The figure shows three views and two pictorial views of one solid part (mm, origin at its lowest corner). Answer the questions. A direction names the side the tool comes from. Round coordinates to 2 decimals unless told otherwise and drop trailing zeros. Order: outer loops, then holes, each group sorted by start corner. A loop starts at its lowest first (then second) coordinate and runs counter-clockwise, first axis right, second up. Notation, with made-up numbers: (9, -15) - (66, -15) arc R32 ccw to (66, 16) - close; hole circle Ø8 at (-29, 33). An arc over 180 degrees is marked (long way). Answer in a Markdown table with one row per item.
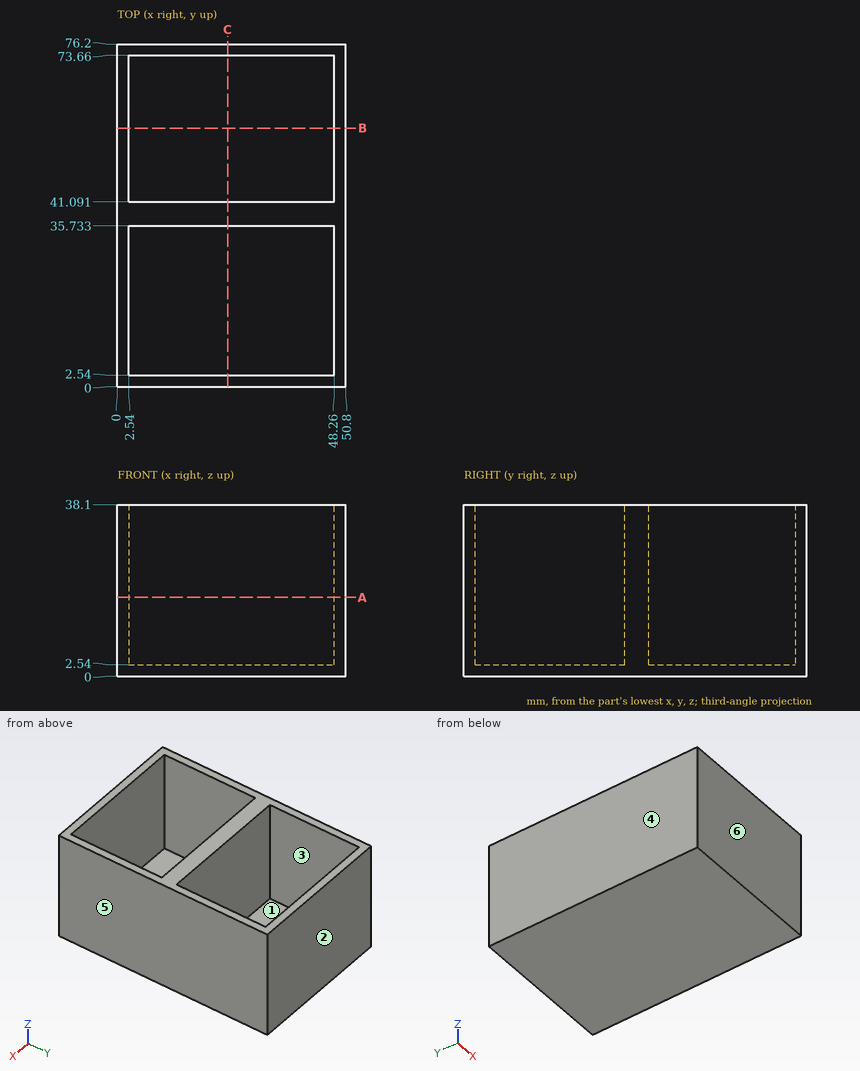
1) Each of these flat-tipped pins is pushed along its axis until it touches: pin 1 (8 mm diameter, centred on y = 40.5, z = 24, fed in from -X); pin 2 (6 mm diameter, centred on x = 34.5, y = 66.5, fed in from +Z). Where does it stop, or does it pass through?
Filled in:
| item | result |
|---|---|
| pin 1 | stops at x = 0 |
| pin 2 | stops at z = 2.54 |
2) Which of the six approach directions +Z, -Z, +X, -X, +Y, -Y give full straight-line access (tool end or side, diameter ignored) to the marked faces 1 and 2?
Filled in:
| item | result |
|---|---|
| face 1 | +Z |
| face 2 | +Z, -Z, +X, -X, +Y |
3) Find section B-B, the plane y = 57.5. Give the vertices of the cut face in (x, z), then the cut area to 3 significant figures.
Filled in:
| item | result |
|---|---|
| outline | (0, 0) - (50.8, 0) - (50.8, 38.1) - (48.26, 38.1) - (48.26, 2.54) - (2.54, 2.54) - (2.54, 38.1) - (0, 38.1) - close |
| area | 310 mm^2 |
4) Find the intervals of material crossed by probe 1 along Y at (x, z) = (24, 30.5); probe 2 along X at (y, z) = (5, 24); probe 3 along Z at (x, y) = (35, 20), in increasing order. Write a range as from..to.
Filled in:
| item | result |
|---|---|
| probe 1 | y = 0..2.54, 35.73..41.09, 73.66..76.2 |
| probe 2 | x = 0..2.54, 48.26..50.8 |
| probe 3 | z = 0..2.54 |
5) The mould has two halves that part along X. Classify the marked faces 3, 4, 5 and 6: released by +X, released by -X, zero draft, split by the parting line, or undercut.
Filled in:
| item | result |
|---|---|
| face 3 | undercut |
| face 4 | released by -X |
| face 5 | released by +X |
| face 6 | zero draft |
6) Find section C-C, the plane x = 24.5. Give the vertices of the cut face in (y, z).
Filled in:
| item | result |
|---|---|
| outline | (0, 0) - (76.2, 0) - (76.2, 38.1) - (73.66, 38.1) - (73.66, 2.54) - (41.09, 2.54) - (41.09, 38.1) - (35.73, 38.1) - (35.73, 2.54) - (2.54, 2.54) - (2.54, 38.1) - (0, 38.1) - close |
7) Find section A-A, the plane z = 17.5. Give the vertices of the cut face in (x, y).
Filled in:
| item | result |
|---|---|
| outline | (0, 0) - (50.8, 0) - (50.8, 76.2) - (0, 76.2) - close; hole (2.54, 2.54) - (48.26, 2.54) - (48.26, 35.73) - (2.54, 35.73) - close; hole (2.54, 41.09) - (48.26, 41.09) - (48.26, 73.66) - (2.54, 73.66) - close |
